from build123d import *

# Parameters (mm, degrees)
BOSS_EXTRUDE1_DEPTH        = 25
SKETCH2_R                  = 25
CUT_EXTRUDE1_DEPTH         = 15
CUT_EXTRUDE3_DEPTH         = 2
CUT_EXTRUDE4_DEPTH         = 20
FILLET1_R                  = 1
SKETCH3_R                  = 11.1125
CUT_EXTRUDE2_DEPTH         = 19.05
CUT_EXTRUDE6_DEPTH         = 315.340579634
M12X1_5_TAPPED_HOLE1_D     = 10.5
M12X1_5_TAPPED_HOLE1_DEPTH = 31.5
M12X1_5_TAPPED_HOLE1_TIP   = 3.15451825
M4X0_7_TAPPED_HOLE1_D      = 3.3
M4X0_7_TAPPED_HOLE1_DEPTH  = 11.5
M4X0_7_TAPPED_HOLE1_TIP    = 0.991420021
M6X1_0_TAPPED_HOLE1_D      = 5
M6X1_0_TAPPED_HOLE1_DEPTH  = 17
M6X1_0_TAPPED_HOLE1_TIP    = 1.502151548
SKETCH24_W                 = 0.2
SKETCH24_H                 = 1.204653058
CUT_EXTRUDE7_DEPTH         = 3


with BuildPart() as part:
    # Sketch1 → Boss-Extrude1 (new body)
    with BuildSketch(Plane.XY):
        with BuildLine():
            Line((109, 280), (141, 280))
            Line((141, 280), (141, 237.308754644))
            ThreePointArc((141, 237.308754644), (140.012193642, 230.350697696), (137.12683548, 223.942497778))
            ThreePointArc((137.12683548, 223.942497778), (78.660042714, 111.502319563), (39.959807706, -9.176805987))
            ThreePointArc((39.959807706, -9.176805987), (0, -41), (-39.959807706, -9.176805987))
            ThreePointArc((-39.959807706, -9.176805987), (-78.660042714, 111.502319563), (-137.12683548, 223.942497778))
            ThreePointArc((-137.12683548, 223.942497778), (-140.012193642, 230.350697696), (-141, 237.308754644))
            Line((-141, 237.308754644), (-141, 280))
            Line((-141, 280), (-109, 280))
            Line((-109, 280), (-109, 244.142135624))
            ThreePointArc((-109, 244.142135624), (-108.238795325, 240.3153013), (-106.071067812, 237.071067812))
            Line((-106.071067812, 237.071067812), (-67.745166004, 198.745166004))
            ThreePointArc((-67.745166004, 198.745166004), (-46.982071679, 184.871709919), (-22.490332008, 180))
            Line((-22.490332008, 180), (22.490332008, 180))
            ThreePointArc((22.490332008, 180), (46.982071679, 184.871709919), (67.745166004, 198.745166004))
            Line((67.745166004, 198.745166004), (106.071067812, 237.071067812))
            ThreePointArc((106.071067812, 237.071067812), (108.238795325, 240.3153013), (109, 244.142135624))
            Line((109, 244.142135624), (109, 280))
        make_face()
    extrude(amount=BOSS_EXTRUDE1_DEPTH)

    # Sketch2 → Cut-Extrude1 (cut)
    with BuildSketch(Plane.XY.offset(25)):
        Circle(SKETCH2_R)
    extrude(amount=-CUT_EXTRUDE1_DEPTH, mode=Mode.SUBTRACT)

    # Sketch4 → Cut-Extrude3 (cut)
    with BuildSketch(Plane.XY.offset(25)):
        with BuildLine():
            Line((-20, 40), (20, 40))
            ThreePointArc((20, 40), (30.606601718, 44.393398282), (35, 55))
            Line((35, 55), (35, 95))
            ThreePointArc((35, 95), (30.606601718, 105.606601718), (20, 110))
            Line((20, 110), (-20, 110))
            ThreePointArc((-20, 110), (-30.606601718, 105.606601718), (-35, 95))
            Line((-35, 95), (-35, 55))
            ThreePointArc((-35, 55), (-30.606601718, 44.393398282), (-20, 40))
        make_face()
    extrude(amount=-CUT_EXTRUDE3_DEPTH, mode=Mode.SUBTRACT)

    # Sketch5 → Cut-Extrude4 (cut)
    with BuildSketch(Plane.XY.offset(25)):
        with BuildLine():
            Line((22.490332008, 174), (12, 174))
            ThreePointArc((12, 174), (6.343145751, 171.656854249), (4, 166))
            Line((4, 166), (4, 126))
            ThreePointArc((4, 126), (6.343145751, 120.343145751), (12, 118))
            Line((12, 118), (20, 118))
            ThreePointArc((20, 118), (36.263455967, 111.263455967), (43, 95))
            Line((43, 95), (43, 78.677414062))
            ThreePointArc((43, 78.677414062), (49.641403556, 70.793619563), (58.538553925, 75.999690268))
            ThreePointArc((58.538553925, 75.999690268), (88.698463192, 148.674821685), (126.248822694, 217.821516145))
            ThreePointArc((126.248822694, 217.821516145), (126.406316455, 225.909739707), (119.426779549, 230))
            Line((119.426779549, 230), (110.798989873, 230))
            ThreePointArc((110.798989873, 230), (107.737522414, 229.39103626), (105.142135624, 227.656854249))
            Line((105.142135624, 227.656854249), (71.987806691, 194.502525317))
            ThreePointArc((71.987806691, 194.502525317), (49.278172274, 179.328432724), (22.490332008, 174))
        make_face()
        with BuildLine():
            Line((-43, 95), (-43, 78.677414062))
            ThreePointArc((-43, 78.677414062), (-49.641403556, 70.793619563), (-58.538553925, 75.999690268))
            ThreePointArc((-58.538553925, 75.999690268), (-88.698463192, 148.674821685), (-126.248822694, 217.821516145))
            ThreePointArc((-126.248822694, 217.821516145), (-126.406316455, 225.909739707), (-119.426779549, 230))
            Line((-119.426779549, 230), (-110.798989873, 230))
            ThreePointArc((-110.798989873, 230), (-107.737522414, 229.39103626), (-105.142135624, 227.656854249))
            Line((-105.142135624, 227.656854249), (-71.987806691, 194.502525317))
            ThreePointArc((-71.987806691, 194.502525317), (-49.278172274, 179.328432724), (-22.490332008, 174))
            Line((-22.490332008, 174), (-12, 174))
            ThreePointArc((-12, 174), (-6.343145751, 171.656854249), (-4, 166))
            Line((-4, 166), (-4, 126))
            ThreePointArc((-4, 126), (-6.343145751, 120.343145751), (-12, 118))
            Line((-12, 118), (-20, 118))
            ThreePointArc((-20, 118), (-36.263455967, 111.263455967), (-43, 95))
        make_face()
    extrude(amount=-CUT_EXTRUDE4_DEPTH, mode=Mode.SUBTRACT)

    # Fillet1
    fillet1_edges = [part.edges().sort_by_distance(p)[0] for p in [
        (78.660042714, 111.502319563, 25),
        (140.012193642, 230.350697696, 25),
        (-140.012193642, 230.350697696, 0),
        (141, 258.654377322, 25),
        (-141, 258.654377322, 0),
        (-125, 280, 0),
        (-109, 262.071067812, 0),
        (-108.238795325, 240.3153013, 0),
        (-86.908116908, 217.908116908, 0),
        (-46.982071679, 184.871709919, 0),
        (0, 180, 0),
        (46.982071679, 184.871709919, 0),
        (125, 280, 25),
        (86.908116908, 217.908116908, 0),
        (108.238795325, 240.3153013, 0),
        (109, 262.071067812, 0),
        (125, 280, 0),
        (141, 258.654377322, 0),
        (140.012193642, 230.350697696, 0),
        (78.660042714, 111.502319563, 0),
        (109, 262.071067812, 25),
        (0, -41, 0),
        (-78.660042714, 111.502319563, 0),
        (108.238795325, 240.3153013, 25),
        (86.908116908, 217.908116908, 25),
        (-141, 280, 12.5),
        (-109, 280, 12.5),
        (109, 280, 12.5),
        (141, 280, 12.5),
        (46.982071679, 184.871709919, 25),
        (0, 180, 25),
        (-46.982071679, 184.871709919, 25),
        (-78.660042714, 111.502319563, 25),
        (-86.908116908, 217.908116908, 25),
        (-108.238795325, 240.3153013, 25),
        (-109, 262.071067812, 25),
        (-125, 280, 25),
        (-141, 258.654377322, 25),
        (-140.012193642, 230.350697696, 25),
        (0, -41, 25),
    ]]
    fillet(fillet1_edges, radius=FILLET1_R)

    # Sketch3 → Cut-Extrude2 (cut)
    with BuildSketch(Plane.XY.offset(10)):
        Circle(SKETCH3_R)
    extrude(amount=-CUT_EXTRUDE2_DEPTH, mode=Mode.SUBTRACT)

    # Sketch10 → Cut-Extrude6 (cut, through all)
    with BuildSketch(Plane.XY.offset(23)):
        with BuildLine():
            Line((15, 60), (15, 90))
            ThreePointArc((15, 90), (13.242640687, 94.242640687), (9, 96))
            Line((9, 96), (-9, 96))
            ThreePointArc((-9, 96), (-13.242640687, 94.242640687), (-15, 90))
            Line((-15, 90), (-15, 60))
            ThreePointArc((-15, 60), (-13.242640687, 55.757359313), (-9, 54))
            Line((-9, 54), (9, 54))
            ThreePointArc((9, 54), (13.242640687, 55.757359313), (15, 60))
        make_face()
    extrude(amount=-CUT_EXTRUDE6_DEPTH, mode=Mode.SUBTRACT)

    # M12x1.5 Tapped Hole1
    with Locations(Plane(origin=(0, 280, 0), x_dir=(1, 0, 0), z_dir=(0, 1, 0))):
        with Locations((-125, -12.5), (125, -12.5)):
            Hole(M12X1_5_TAPPED_HOLE1_D / 2, depth=M12X1_5_TAPPED_HOLE1_DEPTH)
            with Locations((0, 0, -(M12X1_5_TAPPED_HOLE1_DEPTH + M12X1_5_TAPPED_HOLE1_TIP / 2))):  # 118° drill point
                Cone(0, M12X1_5_TAPPED_HOLE1_D / 2, M12X1_5_TAPPED_HOLE1_TIP, mode=Mode.SUBTRACT)

    # M4x0.7 Tapped Hole1
    with Locations(Plane.XY.offset(25)):
        with Locations((-15, -27.5), (25, 25), (-25, 25), (15, -27.5)):
            Hole(M4X0_7_TAPPED_HOLE1_D / 2, depth=M4X0_7_TAPPED_HOLE1_DEPTH)
            with Locations((0, 0, -(M4X0_7_TAPPED_HOLE1_DEPTH + M4X0_7_TAPPED_HOLE1_TIP / 2))):  # 118° drill point
                Cone(0, M4X0_7_TAPPED_HOLE1_D / 2, M4X0_7_TAPPED_HOLE1_TIP, mode=Mode.SUBTRACT)

    # M6x1.0 Tapped Hole1
    with Locations(Plane.XY.offset(23)):
        with Locations((-22.5, 59), (-22.5, 91), (22.5, 91), (22.5, 59)):
            Hole(M6X1_0_TAPPED_HOLE1_D / 2, depth=M6X1_0_TAPPED_HOLE1_DEPTH)
            with Locations((0, 0, -(M6X1_0_TAPPED_HOLE1_DEPTH + M6X1_0_TAPPED_HOLE1_TIP / 2))):  # 118° drill point
                Cone(0, M6X1_0_TAPPED_HOLE1_D / 2, M6X1_0_TAPPED_HOLE1_TIP, mode=Mode.SUBTRACT)

    # Sketch24 → Cut-Extrude7 (cut)
    with BuildSketch(Plane.XY.offset(25)):
        with Locations((0, -41.592326529)):
            Rectangle(SKETCH24_W, SKETCH24_H)
    extrude(amount=-CUT_EXTRUDE7_DEPTH, mode=Mode.SUBTRACT)


solid = part.part
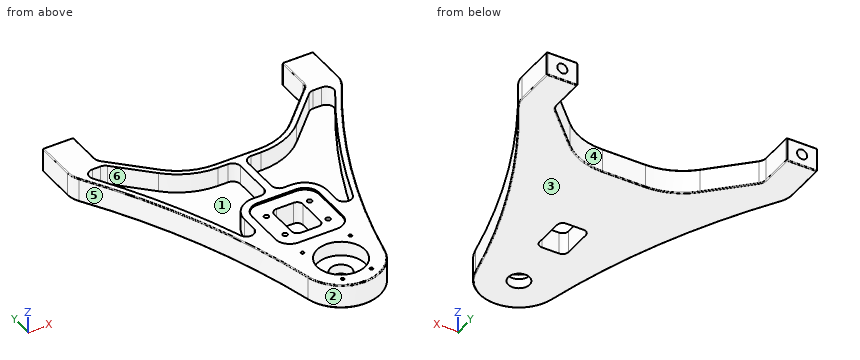
Build history of the part. All positions in model axes, mm. Face numbers are marked on the shaded views. A direction names the side the tool comes from. Coordinates: 2 decimals unless noted, no trailing zeros. One line per item, written item: value.
(1) Probe line 1 (Y direction, x = 0, z = 7.5); line 2 (X direction, y = 155, z = 14); line 3 (X direction, y = 190, z = 5.25). List the from-to ranges inside material, lowest first. Write a range as [from, to].
Checked values:
line 1: [-41, -11.11], [11.11, 54], [96, 180]
line 2: [-98.44, -91.75], [-4, 4], [91.75, 98.44]
line 3: [-116.88, -110.01], [-67.03, -56.84], [56.84, 67.03], [110.01, 116.88]
(2) Drop flat-ended pins along their axis: pin 1 Ø1 at (y, z) = (74, 24) entering from +X; pin 2 Ø11.5 at (x, z) = (-18.5, 12) entering from -Y; pin 3 Ø12 at (x, z) = (35, 21.5) entering from -Y; pin 4 Ø4 at (x, y) = (-27, 184) entering from -Z. Give the stop position or say it passes through.
Checked values:
pin 1: x = 64.37
pin 2: y = -38.97
pin 3: y = -28.98
pin 4: through
(3) Tool access for the marked faces 4, 5 and 6: list every direction of +Z, -Z, +X, -X, +Y, -Y with a clear straight run to the whole face (end or side of a thin tool).
Checked values:
face 4: +Z, -Z, +Y
face 5: +Z, -Z, -X, -Y
face 6: +Z
(4) Mould opens along X. For the marked faces 1, 2 and 3 say: pulls with the +X half, pulls with the -X half, needs draft (parallel to the pull), parting line crosses it, or undercut.
Checked values:
face 1: undercut
face 2: parting line crosses it
face 3: needs draft
